Design review of the part shown in the three views and the two pictorial views. Dimensions are in mm from the part's minimum x, y and z. A direction names the side the tool comes from. Round coordinates to 2 decimals unless told otherwise and drop trailing zeros. Loops run counter-clockwise (first coordinate to the right, second up) from the corner with the lowest first, then second, coordinate; pieces in that order, holes last. Notation, with made-up numbers: M 73,51 L 83,51 A13 cw 83,62 Z; hole C 63.5,61 d11. An arc over 180 degrees is marked long. One line per question, with ' | ' between items.
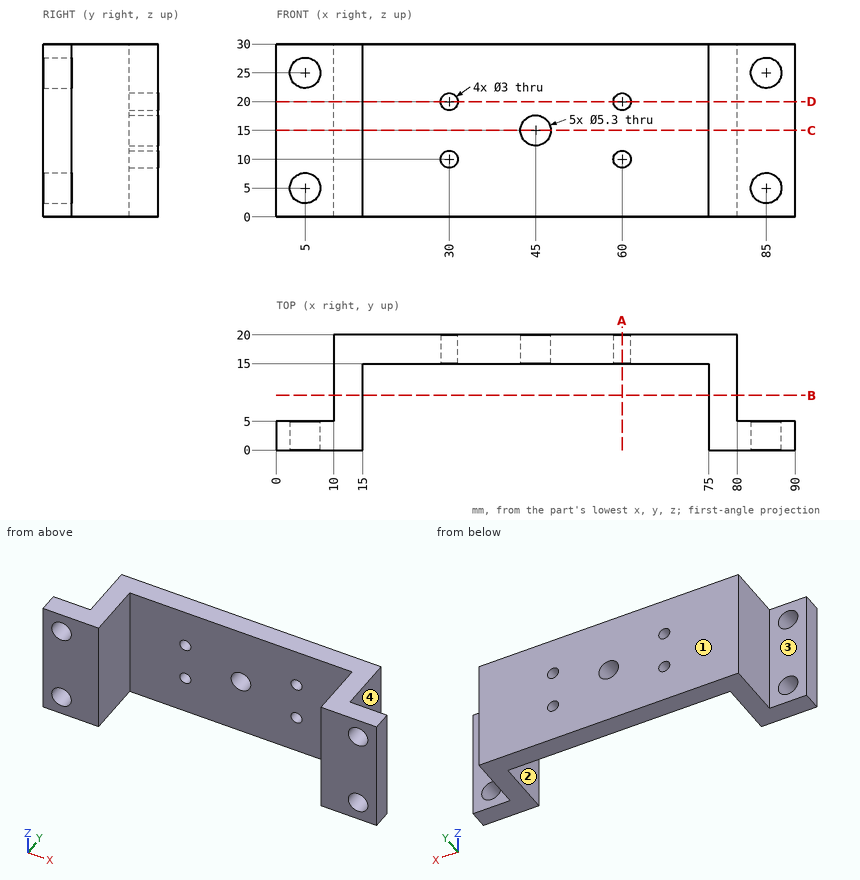
1) Insertion check: P1, Ø12, axis at x = 24.5, y = 5.5, coming from the -Z side; P2, Ø8.5, axis at x = 5, z = 5, coming from the +Y side; P3, Ø12, axis at y = 16, z = 10.5, coming from the -X side. Each pin has a flat end and moves straight along its axis. Give the tip position at first contact, or say it passes through.
Output values:
P1: passes through | P2: stops at y = 5 | P3: stops at x = 10
2) For line 1 (Z direction, x = 30, y = 16.4); line 2 (Z direction, x = 85, y = 3.6); line 3 (Z direction, x = 45, y = 15.5), list the stretches that pass through material, from the lowest coordinate up.
Output values:
line 1: z = 0 to 8.5, 11.5 to 18.5, 21.5 to 30 | line 2: z = 0 to 2.35, 7.65 to 22.35, 27.65 to 30 | line 3: z = 0 to 12.35, 17.65 to 30
3) Add section C-C on z = 15. State the section outline as (x, y) points, then the cut area to 4 significant figures.
Output values:
outline: M 0,0 L 15,0 L 15,15 L 42.35,15 L 42.35,20 L 10,20 L 10,5 L 0,5 Z; M 47.65,15 L 75,15 L 75,0 L 90,0 L 90,5 L 80,5 L 80,20 L 47.65,20 Z | area: 573.5 mm²
4) Add section A-A on x = 60. State the section outline as (y, z) points.
Output values:
outline: M 15,0 L 20,0 L 20,8.5 L 15,8.5 Z; M 15,11.5 L 20,11.5 L 20,18.5 L 15,18.5 Z; M 15,21.5 L 20,21.5 L 20,30 L 15,30 Z
5) Machinability: for the marked faces 1, 2, 3 and 4, which of the approach directions +Z, -Z, +X, -X, +Y, -Y give a long, thin tool a straight path to every point of the face, cutting with its end or side? Answer none if there is none.
Output values:
face 1: +Z, -Z, +X, -X, +Y | face 2: +Z, -Z, -Y | face 3: +Z, -Z, -X, +Y | face 4: +Z, -Z, +X, +Y
6) Add section D-D on z = 20. State the section outline as (x, y) points.
Output values:
outline: M 0,0 L 15,0 L 15,15 L 28.5,15 L 28.5,20 L 10,20 L 10,5 L 0,5 Z; M 31.5,15 L 58.5,15 L 58.5,20 L 31.5,20 Z; M 61.5,15 L 75,15 L 75,0 L 90,0 L 90,5 L 80,5 L 80,20 L 61.5,20 Z
7) Add section B-B on y = 9.5. State the section outline as (x, z) points, then the cut area to 3 significant figures.
Output values:
outline: M 10,0 L 15,0 L 15,30 L 10,30 Z; M 75,0 L 80,0 L 80,30 L 75,30 Z | area: 300 mm²
